Here's how the part is built. I have some questions about the finished solid (model axes, mm). A direction names the side the tool comes from. Round coordinates to 2 decimals unless told otherwise and drop trailing zeros. Write each loop counter-clockwise with the first axis right and the second up, starting at its lowest first coordinate (ties: lowest second). Pieces come first, ordered by that corner, then holes. Notation, with made-up numbers: (71, 62) - (95, 62) arc R26 ccw to (95, 90) - close; hole circle Ø6 at (86, 89). An arc over 180 degrees is marked (long way). One line per item, written item: value. Start each with the question number.
Item 1: Imagine slicing it at A-A, the plane x = 0. Please give me the cut outline in (y, z).
Item 2: Thinking about a two-plate mould opening in X: for faces 1 (the face through (-42.115, 1.62, 31.709)), 2 (the face through (76.4, -17.6, 5.1)), 3 (the face through (-48.09, -1.94, 0.13)), which applies, released by +X, released by -X, zero draft, split by the parting line, or undercut?
Item 3: Imagine slicing it at D-D, the plane z = 12. Please give me the cut outline in (x, y), then the cut area to 3 significant figures.
Item 4: Imagine slicing it at C-C, the plane z = 22.5. Please give me the cut outline in (x, y), then the cut area to 3 significant figures.
Item 5: If I drill on line 1 (Z direction, x = 83, y = 0); line 2 (X direction, y = -24, z = 12); line 3 (Y direction, x = 0, z = 44.5), over which ranges is the centre line in solid material (lowest first)?
Item 6: For faces 4 (the face through (77.3, 17.4, 50.1)), 5 (the face through (30.2, -26.5, 10)), 6 (the face through (39, 0, 10)), 7 (the face through (77, 22.5, 27)), which set-ups out of +Z, -Z, +X, -X, +Y, -Y let a thin tool reach every point of the face, with its end or its side?
Item 7: For P1, Ø10, axis at y = -16.5, z = 52.5, coming from the -X side; P2, Ø1, axis at x = 29.5, y = -21.5, coming from the +Z side; P3, Ø5, axis at x = 48, z = 42.5, coming from the -Y side, each with a flat end and sliding along its axis, tell me the tip position at first contact or that it passes through.
Item 8: Imagine slicing it at B-B, the plane x = 79. Please give me the cut outline in (y, z).
```python
from build123d import *

# Parameters (mm, degrees)
F5_DEPTH = 55
F6_R     = 17.5
F7_DEPTH = 70.5
F8_SIZE  = 10
F9_SIZE  = 2


with BuildPart() as f1:
    # F0 (on Front) → F1 (revolve)
    with BuildSketch(Plane.XZ):
        Polygon((35, 32), (35, 0), (50, 0), (50, 60), (42, 60), (42, 32), align=None)
    revolve(axis=Axis((0, 0, 18.633036), (0, 0, 1)))

    # F2 (on Front) → F3 (revolve, cut)
    with BuildSketch(Plane.XZ):
        Polygon((34.955181, 31.998791), (40, 25), (40, 10), (45, 10), (45, 25), (39.898187, 36.992304), align=None)
    revolve(axis=Axis((0, 0, 12.552274), (0, 0, 1)), mode=Mode.SUBTRACT)

    # F4 (on Top) → F5 (join)
    with BuildSketch(Plane.XY):
        with BuildLine():
            ThreePointArc((42.965102, 22.5), (47.095952, 11.585391), (48.5, 0))
            ThreePointArc((48.5, 0), (47.095952, -11.585391), (42.965102, -22.5))
            Line((42.965102, -22.5), (108.965102, -22.5))
            Line((108.965102, -22.5), (108.965102, 22.5))
            Line((108.965102, 22.5), (42.965102, 22.5))
        make_face()
    extrude(amount=F5_DEPTH)

    # F6 (on face) → F7 (cut)
    with BuildSketch(Plane.YZ.offset(108.965102)):
        with Locations((0, 27.5)):
            Circle(F6_R)
    extrude(amount=-F7_DEPTH, mode=Mode.SUBTRACT)

    # F8
    f8_edges = [f1.edges().sort_by_distance(p)[0] for p in [
        (76.808265, -22.5, 55),
        (76.808265, -22.5, 0),
        (76.808265, 22.5, 55),
        (76.808265, 22.5, 0),
    ]]
    chamfer(f8_edges, length=F8_SIZE)

    # F9
    f9_edges = [f1.edges().sort_by_distance(p)[0] for p in [
        (-50, 0, 60),
        (-42, 0, 60),
        (-35, 0, 0),
        (-50, 0, 0),
    ]]
    chamfer(f9_edges, length=F9_SIZE)


solid = f1.part
```
Values follow:
1. outline: (-50, 2) - (-48, 0) - (-37, 0) - (-35, 2) - (-35, 31.94) - (-40, 25) - (-40, 10) - (-45, 10) - (-45, 25) - (-42, 32.05) - (-42, 58) - (-44, 60) - (-48, 60) - (-50, 58) - close; (35, 2) - (37, 0) - (48, 0) - (50, 2) - (50, 58) - (48, 60) - (44, 60) - (42, 58) - (42, 32.05) - (45, 25) - (45, 10) - (40, 10) - (40, 25) - (35, 31.94) - close
2. face 1: undercut
2. face 2: zero draft
2. face 3: split by the parting line
3. outline: (38.47, -8.12) - (38.47, 8.12) - (39.17, 8.12) arc R40 ccw (long way) to (39.17, -8.12) - close; (44.26, -8.12) arc R45 cw (long way) to (44.26, 8.12) - (108.97, 8.12) - (108.97, 22.5) - (44.65, 22.5) arc R50 ccw (long way) to (44.65, -22.5) - (108.97, -22.5) - (108.97, -8.12) - close; hole circle Ø70 at (0, 0)
3. area: 4,340 mm^2
4. outline: (38.47, -10.97) - (38.47, 10.97) arc R40 ccw (long way) to start; (41.76, -16.77) arc R45 cw (long way) to (41.76, 16.77) - (108.97, 16.77) - (108.97, 22.5) - (44.65, 22.5) arc R50 ccw (long way) to (44.65, -22.5) - (108.97, -22.5) - (108.97, -16.77) - close; hole circle Ø70 at (0, 0)
4. area: 3,200 mm^2
5. line 1: z = 0 to 10, 45 to 55
5. line 2: x = -43.86 to -38.07, -32 to -25.48, 25.48 to 32, 38.07 to 43.86
5. line 3: y = -50 to -42, 42 to 50
6. face 4: +Z, +X, +Y
6. face 5: none
6. face 6: +Z, +X
6. face 7: +Z, -Z, +X, +Y
7. P1: stops at x = -48.66
7. P2: stops at z = 30.54
7. P3: stops at y = -22.5
8. outline: (-22.5, 10) - (-12.5, 0) - (12.5, 0) - (22.5, 10) - (22.5, 45) - (12.5, 55) - (-12.5, 55) - (-22.5, 45) - close; hole circle Ø35 at (0, 27.5)
